Design review of the part shown in the three views and the two pictorial views. Dimensions are in mm from the part's minimum x, y and z. A direction names the side the tool comes from. Coordinates: 2 decimals unless noted, no trailing zeros. Loops run counter-clockwise (first coordinate to the right, second up) from the corner with the lowest first, then second, coordinate; pieces in that order, holes last. Notation, with made-up numbers: (-7, -24) -> (6, -24) arc R14 cw to (6, -1) -> close; hole circle Ø1 at (-31.5, 89.25). An arc over 180 degrees is marked (long way). Answer in a Markdown table with one row per item.
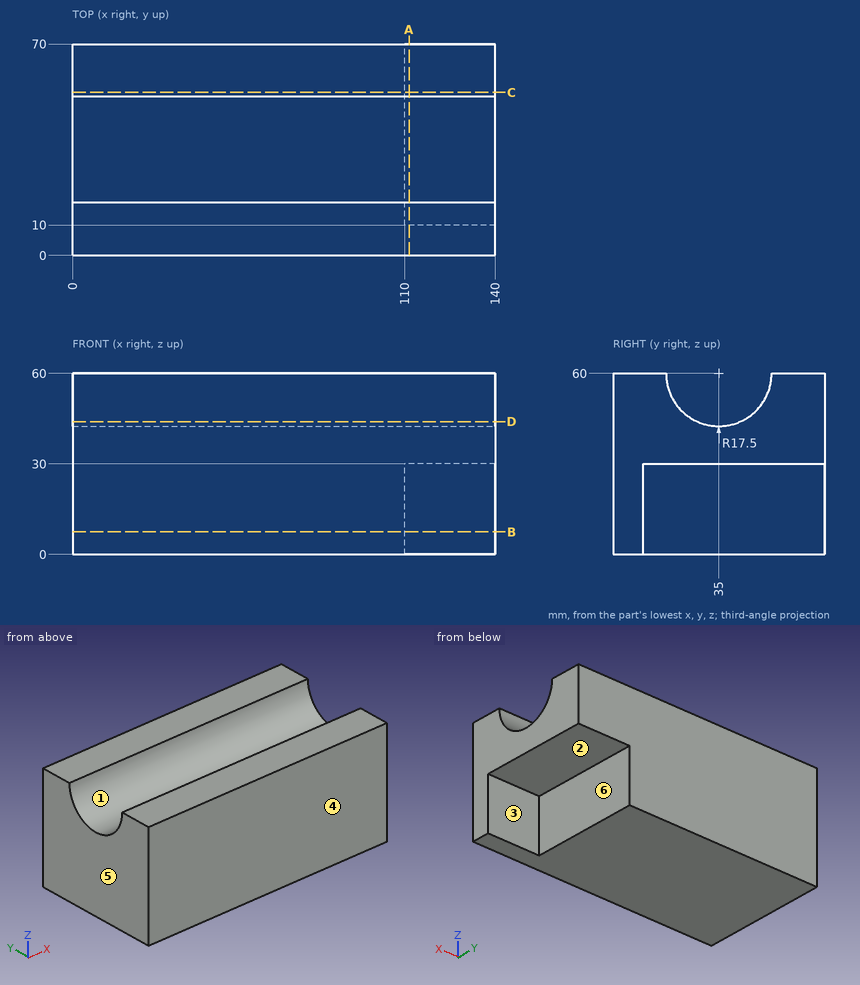
(1) Tool access review of the marked faces 5 and 6: name each direction out of +Z, -Z, +X, -X, +Y, -Y from which nothing blocks a thin tool from reaching the whole face with its end or side.
Evaluation:
| item | result |
|---|---|
| face 5 | +Z, -Z, -X, +Y, -Y |
| face 6 | -Z, +X, +Y |
(2) Take a section at C-C on y = 54. Give the boundary of the cut face in (x, z), and give its area (3 significant figures).
Evaluation:
| item | result |
|---|---|
| outline | (0, 0) -> (110, 0) -> (110, 30) -> (140, 30) -> (140, 60) -> (0, 60) -> close |
| area | 7,500 mm² |
(3) To check wall thickness, follow probe 1 along X at (y, z) = (33.5, 27); probe 2 along Y at (x, z) = (81, 44); probe 3 along Y at (x, z) = (132, 25). State the ranges of each line that lie inside material, in increasing order.
Evaluation:
| item | result |
|---|---|
| probe 1 | x = 0 to 110 |
| probe 2 | y = 0 to 27.91, 42.09 to 70 |
| probe 3 | y = 0 to 10 |
(4) Draft analysis for pull direction Y (two halves, no side actions). For the marked faces 1, 2, 3 and 4, state which applies: pulls with the +Y half, pulls with the -Y half, needs draft (parallel to the pull), parting line crosses it, or undercut.
Evaluation:
| item | result |
|---|---|
| face 1 | undercut |
| face 2 | needs draft |
| face 3 | pulls with the +Y half |
| face 4 | pulls with the -Y half |
(5) Take a section at D-D on z = 44. Give the boundary of the cut face in (x, y), and give its area (3 significant figures).
Evaluation:
| item | result |
|---|---|
| outline | (0, 0) -> (140, 0) -> (140, 27.91) -> (0, 27.91) -> close; (0, 42.09) -> (140, 42.09) -> (140, 70) -> (0, 70) -> close |
| area | 7,820 mm² |
(6) For pin 1 (10 mm diameter, centred on y = 40, z = 16, fed in from +X); pin 2 (4 mm diameter, centred on x = 93, y = 26.5, fed in from +Z), all flat-tipped, find the tip position at first contact; note any pin that passes through.
Evaluation:
| item | result |
|---|---|
| pin 1 | stops at x = 110 |
| pin 2 | stops at z = 46 |
(7) Take a section at A-A on x = 111.5. Give the boundary of the cut face in (y, z), and give its area (3 significant figures).
Evaluation:
| item | result |
|---|---|
| outline | (0, 0) -> (10, 0) -> (10, 30) -> (70, 30) -> (70, 60) -> (52.5, 60) arc R17.5 cw to (17.5, 60) -> (0, 60) -> close |
| area | 1,920 mm² |
(8) Take a section at B-B on z = 7.5. Give the boundary of the cut face in (x, y).
Evaluation:
| item | result |
|---|---|
| outline | (0, 0) -> (140, 0) -> (140, 10) -> (110, 10) -> (110, 70) -> (0, 70) -> close |
